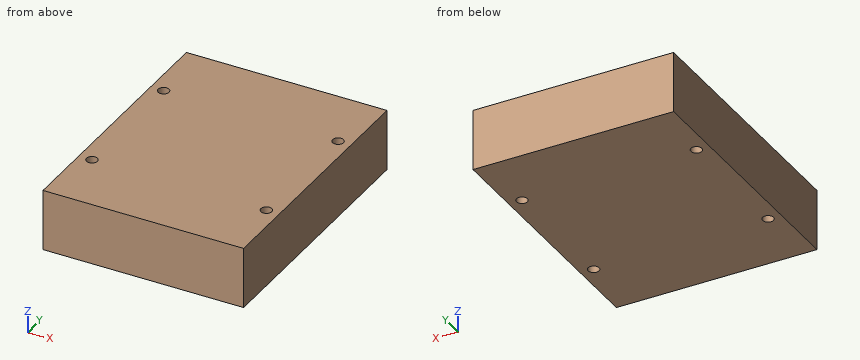
Solid Edge part; units mm, degrees
sketch "Sketch1" plane through (0, 0, 0) normal (0, 0, 1) x (1, 0, 0)
  line L0 (-29.21, 38.1) -> (29.21, 38.1)
  line L1 (29.21, 38.1) -> (29.21, -38.1)
  line L2 (29.21, -38.1) -> (-29.21, -38.1)
  line L3 (-29.21, -38.1) -> (-29.21, 38.1)
  dimension "D1" = 29.21
  dimension "D2" = 29.21
extrude "Protrusion1" add sketch "Sketch1" along normal blind 17.78
hole "Hole_1" at (25.4, 19.05, 17.78) direction (0, 0, -1) diameter 3.175 end up to next
hole "Hole1" at (25.4, -19.05, 17.78) direction (0, 0, -1) diameter 3.175 end up to next
hole "Hole2" at (-25.4, -19.05, 17.78) direction (0, 0, -1) diameter 3.175 end up to next
hole "Hole3" at (-25.4, 19.05, 17.78) direction (0, 0, -1) diameter 3.175 end up to next
CAD build for the part. Positions are in the model's coordinates, mm. Round coordinates to 2 decimals unless told otherwise and drop trailing zeros. Write each loop counter-clockwise with the first axis right and the second up, starting at its lowest first coordinate (ties: lowest second). Pieces come first, ordered by that corner, then holes.
(1) Probe line 1 along X through (y, z) = (19.05, 12.75); line 2 along Y through (x, z) = (25.4, 5.5); line 3 along X through (y, z) = (18.5, 16.5). List the from-to ranges inside material, lowest first.
(2) Drop flat-ended pins along their axis: P1, Ø2.5, axis at x = 25.4, y = 19.05, coming from the +Z side; P2, Ø5, axis at x = 25.4, y = -19.05, coming from the +Z side. Give the stop position or say it passes through.
(3) Slice it at B-B, the plane y = 19.05. Write the cut outline in (x, z).
(4) Slice it at A-A, the plane x = -25.4. Write the cut outline in (y, z).
From the geometry:
1. line 1: x = -29.21 to -26.99, -23.81 to 23.81, 26.99 to 29.21
1. line 2: y = -38.1 to -20.64, -17.46 to 17.46, 20.64 to 38.1
1. line 3: x = -29.21 to -26.89, -23.91 to 23.91, 26.89 to 29.21
2. P1: passes through
2. P2: stops at z = 17.78
3. outline: (-29.21, 0) - (-26.99, 0) - (-26.99, 17.78) - (-29.21, 17.78) - close; (-23.81, 0) - (23.81, 0) - (23.81, 17.78) - (-23.81, 17.78) - close; (26.99, 0) - (29.21, 0) - (29.21, 17.78) - (26.99, 17.78) - close
4. outline: (-38.1, 0) - (-20.64, 0) - (-20.64, 17.78) - (-38.1, 17.78) - close; (-17.46, 0) - (17.46, 0) - (17.46, 17.78) - (-17.46, 17.78) - close; (20.64, 0) - (38.1, 0) - (38.1, 17.78) - (20.64, 17.78) - close
